Work out the finished part from the listing and answer in its coordinate system (mm). Face numbers are marked on the shaded views. A direction names the side the tool comes from. Round coordinates to 2 decimals unless told otherwise and drop trailing zeros. Order: outer loops, then holes, each group sorted by start corner. A loop starts at its lowest first (then second) coordinate and runs counter-clockwise, first axis right, second up. Notation, with made-up numbers: (-8, 62.25) -> (17, 62.25) arc R20 ccw to (17, 81.25) -> close; hole circle Ø2 at (74, 46). An arc over 180 degrees is marked (long way). Use a Markdown table: item, result. Add a question column.
Item 1: Flat-ended cylindrical pins translate along their axes: P1, Ø2, axis at y = 10.5, z = 4.5, coming from the +X side; P2, Ø10, axis at x = -11, y = 2.5, coming from the +Z side; P3, Ø1, axis at x = -4.5, z = 0, coming from the +Y side. Find the tip coordinate at first contact, or state that the pin passes through.
Item 2: A cutting plane is placed at C-C, the plane z = 9.5. Determine the outline of the cut face in (x, y), plus the area to 3 significant figures.
Item 3: Find the intervals of material crossed by L1, parallel to Y at x = 0, z = 1.05; L2, parallel to Z at x = 7.25, y = -11; L3, parallel to Z at x = -6.5, y = -2.25, in increasing order. Write a range as [from, to].
Item 4: A tool of negligible diameter and unlimited length cuts with its end or side. For the marked faces 4, 5 and 6, from which of +Z, -Z, +X, -X, +Y, -Y can it reach the whole face along a straight path? Write none if from no direction.
Item 5: A cutting plane is placed at B-B, the plane z = 1.5. Determine the outline of the cut face in (x, y), plus the area to 3 significant figures.
Item 6: A cutting plane is placed at A-A, the plane z = 6.5. Determine the outline of the cut face in (x, y), plus the area to 3 significant figures.
Item 7: For a pull along X with two mould halves and no side action, classify the marked faces 1, 2 and 3 as +X half, -X half, draft (parallel to the pull), parting line (faces both ways), or undercut.
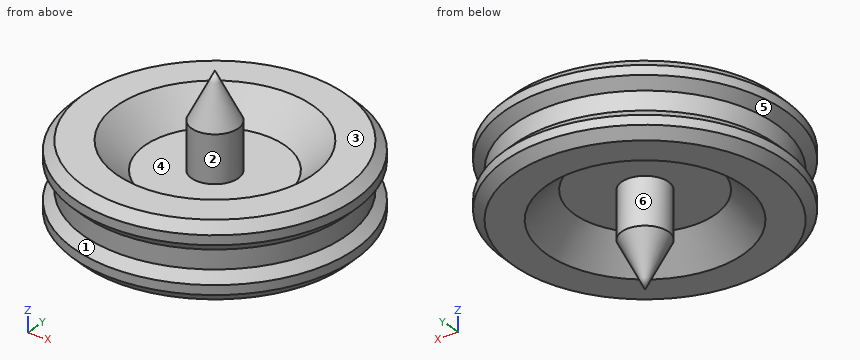
from build123d import *

# Parameters (mm, degrees)
F0_R     = 14
F1_DEPTH = 1
F2_R     = 15
F2_R_2   = 14
F2_R_3   = 7.5
F3_DEPTH = 3
F2_R_4   = 2.5
F4_DEPTH = 10
F5_SIZE  = 0.99999
F6_SIZE  = 2.99999
F7_SIZE2 = 5
F7_SIZE  = 2.5


# Not quite as in the source:
# - a fillet or chamfer is up to 0.001 mm smaller than in the source, because OpenCascade refuses the exact size


with BuildPart() as f1:
    # F0 (on Top) → F1 (new body)
    with BuildSketch(Plane.XY):
        Circle(F0_R)
    extrude(amount=F1_DEPTH)

    # F2 (on face) → F3 (join)
    with BuildSketch(Plane.XY.offset(1)):
        Circle(F2_R)
        Circle(F2_R_2, mode=Mode.SUBTRACT)
        Circle(F2_R_2)
        Circle(F2_R_3, mode=Mode.SUBTRACT)
    extrude(amount=F3_DEPTH)

    # F2 (on face) → F4 (join)
    with BuildSketch(Plane.XY.offset(1)):
        Circle(F2_R_4)
    extrude(amount=F4_DEPTH)

    # F5 (size 1 in the source; OpenCascade refuses exactly that, so slightly less here)
    f5_edges = [f1.edges().sort_by_distance(p)[0] for p in [
        (-15, 0, 4),
        (-15, 0, 1),
    ]]
    chamfer(f5_edges, length=F5_SIZE)

    # F6 (size 3 in the source; OpenCascade refuses exactly that, so slightly less here)
    f6_edges = [f1.edges().sort_by_distance(p)[0] for p in [
        (-7.5, 0, 4),
    ]]
    chamfer(f6_edges, length=F6_SIZE)

    # F7
    f7_edges = [f1.edges().sort_by_distance(p)[0] for p in [
        (-2.5, 0, 11),
    ]]
    f7_side = f1.faces().sort_by_distance((0, 0, 11))[0]
    chamfer(f7_edges, length=F7_SIZE, length2=F7_SIZE2, reference=f7_side)

    # F8: F1 across plane


with BuildPart() as f1_1:
    add(f1.part)
    add(f1.part.mirror(Plane.XY))


solid = f1_1.part
Reported:
| question | item | result |
|---|---|---|
| 1 | P1 | x = 10.32 |
| 1 | P2 | z = 4 |
| 1 | P3 | y = 13.42 |
| 2 | outline | circle Ø1.5 at (0, 0) |
| 2 | area | 1.77 mm² |
| 3 | L1 | [-14.05, -7.55], [-2.5, 2.5], [7.55, 14.05] |
| 3 | L2 | [-4, 4] |
| 3 | L3 | [-1, 1] |
| 4 | face 4 | +Z |
| 4 | face 5 | none |
| 4 | face 6 | -Z |
| 5 | outline | circle Ø29 at (0, 0); circle Ø5 at (0, 0); hole circle Ø16 at (0, 0) |
| 5 | area | 479 mm² |
| 6 | outline | circle Ø4.5 at (0, 0) |
| 6 | area | 15.9 mm² |
| 7 | face 1 | parting line |
| 7 | face 2 | undercut |
| 7 | face 3 | draft |
